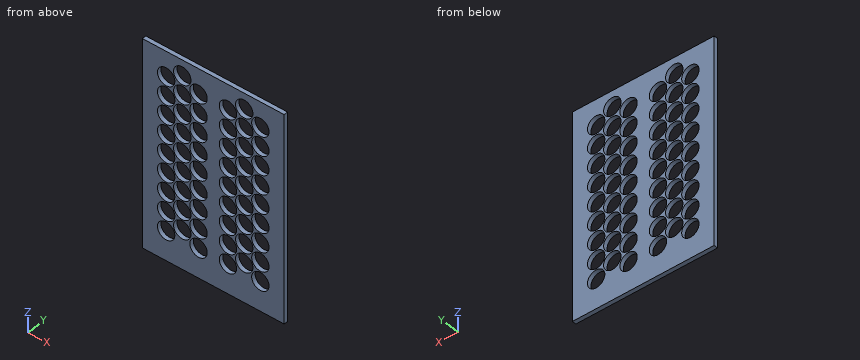
```python
from build123d import *

# Parameters (mm, degrees)
SKETCH1_W           = 177.8
SKETCH1_H           = 254
SKETCH1_R           = 10.90200004
BOSS_EXTRUDE1_DEPTH = 5.08


with BuildPart() as part:
    # Sketch1 → Boss-Extrude1 (new body)
    with BuildSketch(Plane(origin=(0, 0, 0), x_dir=(1, 0, 0), z_dir=(0, 1, 0))):
        Rectangle(SKETCH1_W, SKETCH1_H)
        with Locations(Location((-59.07499996, 90.82499996, 0), (0, 0, 270))):
            Circle(SKETCH1_R, mode=Mode.SUBTRACT)
        with Locations(Location((-18.43499996, 90.82499996, 0), (0, 0, 270))):
            Circle(SKETCH1_R, mode=Mode.SUBTRACT)
        with Locations(Location((-18.43499996, 67.45699996, 0), (0, 0, 270))):
            Circle(SKETCH1_R, mode=Mode.SUBTRACT)
        with Locations(Location((-18.43499996, 44.08899996, 0), (0, 0, 270))):
            Circle(SKETCH1_R, mode=Mode.SUBTRACT)
        with Locations(Location((-18.43499996, 20.72099996, 0), (0, 0, 270))):
            Circle(SKETCH1_R, mode=Mode.SUBTRACT)
        with Locations(Location((-18.43499996, -2.64700004, 0), (0, 0, 270))):
            Circle(SKETCH1_R, mode=Mode.SUBTRACT)
        with Locations(Location((-18.43499996, -26.01500004, 0), (0, 0, 270))):
            Circle(SKETCH1_R, mode=Mode.SUBTRACT)
        with Locations(Location((-18.43499996, -49.38300004, 0), (0, 0, 270))):
            Circle(SKETCH1_R, mode=Mode.SUBTRACT)
        with Locations(Location((-18.43499996, -72.75100004, 0), (0, 0, 270))):
            Circle(SKETCH1_R, mode=Mode.SUBTRACT)
        with Locations(Location((-18.43499996, -96.11900004, 0), (0, 0, 270))):
            Circle(SKETCH1_R, mode=Mode.SUBTRACT)
        with Locations(Location((-59.07499996, 67.45699996, 0), (0, 0, 270))):
            Circle(SKETCH1_R, mode=Mode.SUBTRACT)
        with Locations(Location((-59.07499996, 44.08899996, 0), (0, 0, 270))):
            Circle(SKETCH1_R, mode=Mode.SUBTRACT)
        with Locations(Location((-59.07499996, 20.72099996, 0), (0, 0, 270))):
            Circle(SKETCH1_R, mode=Mode.SUBTRACT)
        with Locations(Location((-59.07499996, -2.64700004, 0), (0, 0, 270))):
            Circle(SKETCH1_R, mode=Mode.SUBTRACT)
        with Locations(Location((-59.07499996, -26.01500004, 0), (0, 0, 270))):
            Circle(SKETCH1_R, mode=Mode.SUBTRACT)
        with Locations(Location((-59.07499996, -49.38300004, 0), (0, 0, 270))):
            Circle(SKETCH1_R, mode=Mode.SUBTRACT)
        with Locations(Location((-59.07499996, -72.75100004, 0), (0, 0, 270))):
            Circle(SKETCH1_R, mode=Mode.SUBTRACT)
        with Locations(Location((-59.07499996, -96.11900004, 0), (0, 0, 270))):
            Circle(SKETCH1_R, mode=Mode.SUBTRACT)
        with Locations(Location((-38.837718324, -107.80300004, 0), (0, 0, 270))):
            Circle(SKETCH1_R, mode=Mode.SUBTRACT)
        with Locations(Location((-38.837718324, -84.43500004, 0), (0, 0, 270))):
            Circle(SKETCH1_R, mode=Mode.SUBTRACT)
        with Locations(Location((-38.837718324, -61.06700004, 0), (0, 0, 270))):
            Circle(SKETCH1_R, mode=Mode.SUBTRACT)
        with Locations(Location((-38.837718324, -37.69900004, 0), (0, 0, 270))):
            Circle(SKETCH1_R, mode=Mode.SUBTRACT)
        with Locations(Location((-38.837718324, -14.33100004, 0), (0, 0, 270))):
            Circle(SKETCH1_R, mode=Mode.SUBTRACT)
        with Locations(Location((-38.837718324, 9.03699996, 0), (0, 0, 270))):
            Circle(SKETCH1_R, mode=Mode.SUBTRACT)
        with Locations(Location((-38.837718324, 32.40499996, 0), (0, 0, 270))):
            Circle(SKETCH1_R, mode=Mode.SUBTRACT)
        with Locations(Location((-38.837718324, 55.77299996, 0), (0, 0, 270))):
            Circle(SKETCH1_R, mode=Mode.SUBTRACT)
        with Locations(Location((-38.837718324, 79.14099996, 0), (0, 0, 270))):
            Circle(SKETCH1_R, mode=Mode.SUBTRACT)
        with Locations(Location((59.07499996, -96.11900004, 0), (0, 0, 90))):
            Circle(SKETCH1_R, mode=Mode.SUBTRACT)
        with Locations(Location((18.43499996, -72.75100004, 0), (0, 0, 90))):
            Circle(SKETCH1_R, mode=Mode.SUBTRACT)
        with Locations(Location((18.43499996, -96.11900004, 0), (0, 0, 90))):
            Circle(SKETCH1_R, mode=Mode.SUBTRACT)
        with Locations(Location((38.837718324, -84.43500004, 0), (0, 0, 90))):
            Circle(SKETCH1_R, mode=Mode.SUBTRACT)
        with Locations(Location((38.837718324, -107.80300004, 0), (0, 0, 90))):
            Circle(SKETCH1_R, mode=Mode.SUBTRACT)
        with Locations(Location((59.07499996, -72.75100004, 0), (0, 0, 90))):
            Circle(SKETCH1_R, mode=Mode.SUBTRACT)
        with Locations(Location((59.07499996, -49.38300004, 0), (0, 0, 90))):
            Circle(SKETCH1_R, mode=Mode.SUBTRACT)
        with Locations(Location((38.837718324, -61.06700004, 0), (0, 0, 90))):
            Circle(SKETCH1_R, mode=Mode.SUBTRACT)
        with Locations(Location((18.43499996, -49.38300004, 0), (0, 0, 90))):
            Circle(SKETCH1_R, mode=Mode.SUBTRACT)
        with Locations(Location((38.837718324, -37.69900004, 0), (0, 0, 90))):
            Circle(SKETCH1_R, mode=Mode.SUBTRACT)
        with Locations(Location((59.07499996, -26.01500004, 0), (0, 0, 90))):
            Circle(SKETCH1_R, mode=Mode.SUBTRACT)
        with Locations(Location((18.43499996, -26.01500004, 0), (0, 0, 90))):
            Circle(SKETCH1_R, mode=Mode.SUBTRACT)
        with Locations(Location((38.837718324, -14.33100004, 0), (0, 0, 90))):
            Circle(SKETCH1_R, mode=Mode.SUBTRACT)
        with Locations(Location((59.07499996, -2.64700004, 0), (0, 0, 90))):
            Circle(SKETCH1_R, mode=Mode.SUBTRACT)
        with Locations(Location((18.43499996, -2.64700004, 0), (0, 0, 90))):
            Circle(SKETCH1_R, mode=Mode.SUBTRACT)
        with Locations(Location((38.837718324, 9.03699996, 0), (0, 0, 90))):
            Circle(SKETCH1_R, mode=Mode.SUBTRACT)
        with Locations(Location((59.07499996, 20.72099996, 0), (0, 0, 90))):
            Circle(SKETCH1_R, mode=Mode.SUBTRACT)
        with Locations(Location((18.43499996, 20.72099996, 0), (0, 0, 90))):
            Circle(SKETCH1_R, mode=Mode.SUBTRACT)
        with Locations(Location((38.837718324, 32.40499996, 0), (0, 0, 90))):
            Circle(SKETCH1_R, mode=Mode.SUBTRACT)
        with Locations(Location((59.07499996, 44.08899996, 0), (0, 0, 90))):
            Circle(SKETCH1_R, mode=Mode.SUBTRACT)
        with Locations(Location((18.43499996, 44.08899996, 0), (0, 0, 90))):
            Circle(SKETCH1_R, mode=Mode.SUBTRACT)
        with Locations(Location((18.43499996, 67.45699996, 0), (0, 0, 90))):
            Circle(SKETCH1_R, mode=Mode.SUBTRACT)
        with Locations(Location((38.837718324, 55.77299996, 0), (0, 0, 90))):
            Circle(SKETCH1_R, mode=Mode.SUBTRACT)
        with Locations(Location((59.07499996, 67.45699996, 0), (0, 0, 90))):
            Circle(SKETCH1_R, mode=Mode.SUBTRACT)
        with Locations(Location((38.837718324, 79.14099996, 0), (0, 0, 90))):
            Circle(SKETCH1_R, mode=Mode.SUBTRACT)
        with Locations(Location((18.43499996, 90.82499996, 0), (0, 0, 90))):
            Circle(SKETCH1_R, mode=Mode.SUBTRACT)
        with Locations(Location((59.07499996, 90.82499996, 0), (0, 0, 90))):
            Circle(SKETCH1_R, mode=Mode.SUBTRACT)
    extrude(amount=BOSS_EXTRUDE1_DEPTH)


solid = part.part
```
Check sheet for the modelled part. Datum: model origin and axes. Units: mm. Give positions to 0.01 mm unless a question says otherwise; leave off trailing zeros. Loops run counter-clockwise (first coordinate to the right, second up) from the corner with the lowest first, then second, coordinate; pieces in that order, holes last. Notation, with made-up numbers: (11, 0) - (53, 0) arc R22 ccw to (53, 20) - close; hole circle Ø5 at (46, 13). An arc over 180 degrees is marked (long way). One line per question, with ' | ' between items. Start each with the question number.
1. Cross-section at A-A, the plane z = 44.5. Enter the section's corners in (x, y).
2. Cross-section at D-D, the plane z = -40. Enter the section's corners in (x, y).
3. Material ranges on line 1 along X through (y, z) = (1.3, 96); line 2 along X through (y, z) = (4.65, -93), recorded low to high. Write a range as [from, to].
4. Cross-section at B-B, the plane x = -22. Give the number of separate pieces and of enclosed holes in the cut face, plus the area to 3 significant figures.
Check result:
1) outline: (-88.9, 0) - (-68.82, 0) - (-68.82, 5.08) - (-88.9, 5.08) - close; (-49.33, 0) - (-47.36, 0) - (-47.36, 5.08) - (-49.33, 5.08) - close; (-30.32, 0) - (-28.18, 0) - (-28.18, 5.08) - (-30.32, 5.08) - close; (-8.69, 0) - (8.69, 0) - (8.69, 5.08) - (-8.69, 5.08) - close; (28.18, 0) - (30.32, 0) - (30.32, 5.08) - (28.18, 5.08) - close; (47.36, 0) - (49.33, 0) - (49.33, 5.08) - (47.36, 5.08) - close; (68.82, 0) - (88.9, 0) - (88.9, 5.08) - (68.82, 5.08) - close
2) outline: (-88.9, 0) - (-69.18, 0) - (-69.18, 5.08) - (-88.9, 5.08) - close; (-48.97, 0) - (-46.66, 0) - (-46.66, 5.08) - (-48.97, 5.08) - close; (-31.02, 0) - (-28.54, 0) - (-28.54, 5.08) - (-31.02, 5.08) - close; (-8.33, 0) - (8.33, 0) - (8.33, 5.08) - (-8.33, 5.08) - close; (28.54, 0) - (31.02, 0) - (31.02, 5.08) - (28.54, 5.08) - close; (46.66, 0) - (48.97, 0) - (48.97, 5.08) - (46.66, 5.08) - close; (69.18, 0) - (88.9, 0) - (88.9, 5.08) - (69.18, 5.08) - close
3) line 1: x = [-88.9, -69.98], [-48.17, -29.34], [-7.53, 7.53], [29.34, 48.17], [69.98, 88.9] | line 2: x = [-88.9, -69.76], [-48.39, -29.12], [-7.75, 7.75], [29.12, 48.39], [69.76, 88.9]
4) separate pieces: 10 | enclosed holes: 0 | area: 348 mm2
